Work out the finished part from the listing and answer in its coordinate system (mm). A direction names the side the tool comes from. Give positions to 0.01 mm unless a question says otherwise; leave off trailing zeros. Loops run counter-clockwise (first coordinate to the right, second up) from the corner with the lowest first, then second, coordinate; pieces in that order, holes last. Notation, with made-up numbers: (85.25, 9.25) - (92.25, 9.25) arc R22 cw to (92.25, 37.25) - close; hole circle Ø4 at (5, 77.25). An arc over 180 degrees is marked (long way). Use CSV: the item, a comma, the result in double quotes.
from build123d import *

# Parameters (mm, degrees)
BOSS_EXTRUDE1_DEPTH   = 5
SKETCH2_R             = 1.75
LUKNE_M3_VIJAKI_DEPTH = 5
SKETCH3_W             = 80
SKETCH3_H             = 73
CUT_EXTRUDE2_DEPTH    = 5


with BuildPart() as part:
    # Sketch1 → Boss-Extrude1 (new body)
    with BuildSketch(Plane.XY):
        with BuildLine():
            Line((-115, -60), (115, -60))
            ThreePointArc((115, -60), (118.535533906, -58.535533906), (120, -55))
            Line((120, -55), (120, 55))
            ThreePointArc((120, 55), (118.535533906, 58.535533906), (115, 60))
            Line((115, 60), (-115, 60))
            ThreePointArc((-115, 60), (-118.535533906, 58.535533906), (-120, 55))
            Line((-120, 55), (-120, -55))
            ThreePointArc((-120, -55), (-118.535533906, -58.535533906), (-115, -60))
        make_face()
    extrude(amount=BOSS_EXTRUDE1_DEPTH)

    # Sketch2 → lukne_m3_vijaki (cut)
    with BuildSketch(Plane.XY.offset(5)):
        with Locations((-115, 55)):
            Circle(SKETCH2_R)
        with Locations((115, 55)):
            Circle(SKETCH2_R)
        with Locations((115, -55)):
            Circle(SKETCH2_R)
        with Locations((-115, -55)):
            Circle(SKETCH2_R)
    extrude(amount=-LUKNE_M3_VIJAKI_DEPTH, mode=Mode.SUBTRACT)

    # Sketch3 → Cut-Extrude2 (cut)
    with BuildSketch(Plane.XY.offset(5)):
        with Locations((72.5, 13.5)):
            Rectangle(SKETCH3_W, SKETCH3_H)
    extrude(amount=-CUT_EXTRUDE2_DEPTH, mode=Mode.SUBTRACT)


solid = part.part
Item 1: For faces 1 (the flat face through (72, -23, 3)), 2 (the flat face through (-28, 1, 5)), determine the directions among +Z, -Z, +X, -X, +Y, -Y from which every point of the face is accessible in a straight line to the end or side of a thin tool.
Determined:
face 1,"+Z, -Z"
face 2,"+Z, +X, -X, +Y, -Y"
Item 2: A cutting plane is placed at A-A on x = 78. Determine the outline of the cut face in (y, z).
Determined:
outline,"(-60, 0) - (-23, 0) - (-23, 5) - (-60, 5) - close; (50, 0) - (60, 0) - (60, 5) - (50, 5) - close"
Item 3: Find the intervals of material crossed by line 1 (Y direction, x = 115, z = 2.9); line 2 (X direction, y = 4.5, z = 4.6); line 3 (Y direction, x = 60, z = 3), in increasing order.
Determined:
line 1,"y = -60 to -56.75, -53.25 to 53.25, 56.75 to 60"
line 2,"x = -120 to 32.5, 112.5 to 120"
line 3,"y = -60 to -23, 50 to 60"
Item 4: The mould has two halves that part along Y. Classify faces 3 (the flat face through (2, 60, 2)), 4 (the flat face through (72, 50, 3)), 5 (the flat face through (-2, -60, 2)), 6 (the flat face through (112.5, 13, 3)): pulls with the +Y half, pulls with the -Y half, needs draft (parallel to the pull), parting line crosses it, or undercut.
Determined:
face 3,"pulls with the +Y half"
face 4,"undercut"
face 5,"pulls with the -Y half"
face 6,"undercut"
Item 5: A cutting plane is placed at C-C on z = 3.25. Determine the outline of the cut face in (x, y).
Determined:
outline,"(-120, -55) arc R5 ccw to (-115, -60) - (115, -60) arc R5 ccw to (120, -55) - (120, 55) arc R5 ccw to (115, 60) - (-115, 60) arc R5 ccw to (-120, 55) - close; hole circle Ø3.5 at (-115, -55); hole circle Ø3.5 at (-115, 55); hole (32.5, -23) - (112.5, -23) - (112.5, 50) - (32.5, 50) - close; hole circle Ø3.5 at (115, -55); hole circle Ø3.5 at (115, 55)"
Item 6: A cutting plane is placed at B-B on y = 46. Determine the outline of the cut face in (x, z), and give its area (3 significant figures).
Determined:
outline,"(-120, 0) - (32.5, 0) - (32.5, 5) - (-120, 5) - close; (112.5, 0) - (120, 0) - (120, 5) - (112.5, 5) - close"
area,"800 mm²"
